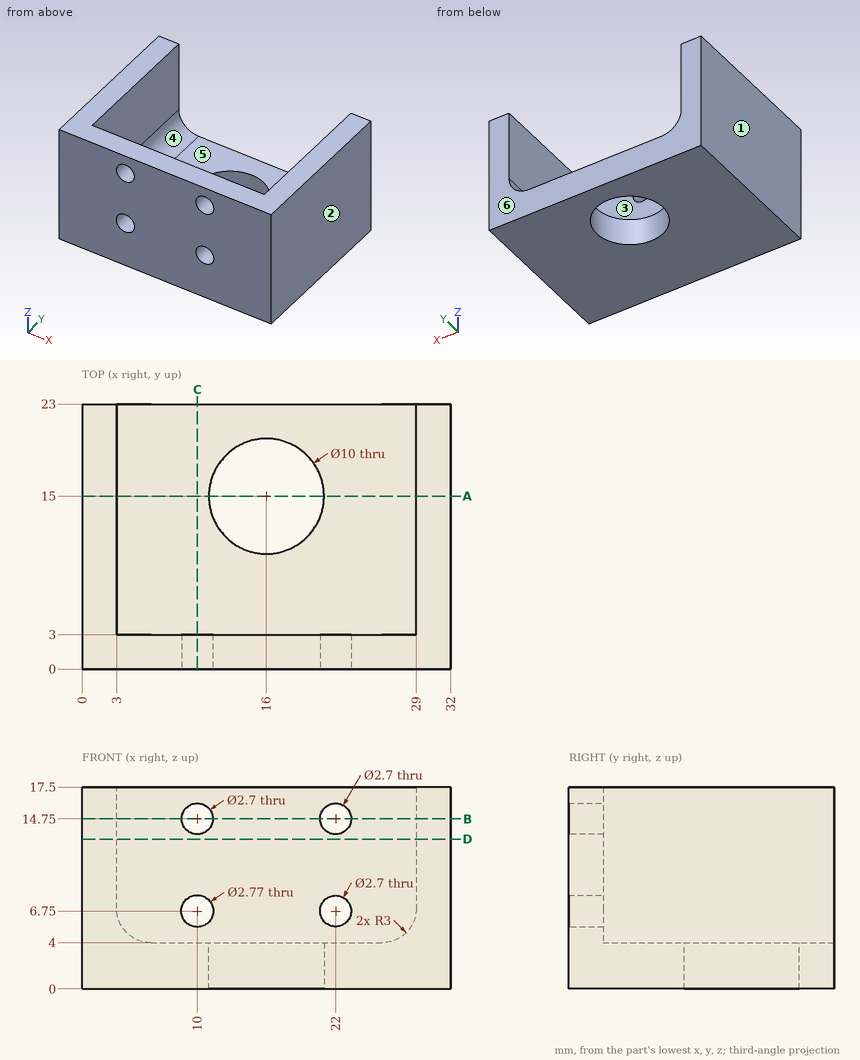
Here's the drawing with two shaded views (mm, measured from the low corner). I have some questions. A direction names the side the tool comes from. Coordinates: 2 decimals unless noted, no trailing zeros. Order: outer loops, then holes, each group sorted by start corner. A loop starts at its lowest first (then second) coordinate and runs counter-clockwise, first axis right, second up.
Item 1: For the marked faces 5 and 6, which set-ups out of +Z, -Z, +X, -X, +Y, -Y let a thin tool reach every point of the face, with its end or its side?
Result sheet:
face 5: +Z, +Y
face 6: +Z, -Z, +X, -X, +Y
Item 2: If we section it at C-C on x = 10: List the corners of the cut face in (y, z) for me (3 decimals), plus the area to 3 significant figures.
Result sheet:
outline: (0, 0) - (23, 0) - (23, 4) - (3, 4) - (3, 5.365) - (0, 5.365) - close; (0, 8.135) - (3, 8.135) - (3, 13.4) - (0, 13.4) - close; (0, 16.1) - (3, 16.1) - (3, 17.5) - (0, 17.5) - close
area: 116 mm2
Item 3: If we section it at B-B on z = 14.75: List the corners of the cut face in (x, y) for me.
Result sheet:
outline: (0, 0) - (8.65, 0) - (8.65, 3) - (3, 3) - (3, 23) - (0, 23) - close; (11.35, 0) - (20.65, 0) - (20.65, 3) - (11.35, 3) - close; (23.35, 0) - (32, 0) - (32, 23) - (29, 23) - (29, 3) - (23.35, 3) - close
Item 4: If we section it at A-A on y = 15: List the corners of the cut face in (x, z) for me.
Result sheet:
outline: (0, 0) - (11, 0) - (11, 4) - (6, 4) arc R3 cw to (3, 7) - (3, 17.5) - (0, 17.5) - close; (21, 0) - (32, 0) - (32, 17.5) - (29, 17.5) - (29, 7) arc R3 cw to (26, 4) - (21, 4) - close
Item 5: For P1, Ø6, axis at x = 16, y = 15, coming from the +Z side; P2, Ø4, axis at x = 21.5, z = 9, coming from the +Y side, each with a flat end and sliding along its axis, tell me the tip position at first contact or that it passes through.
Result sheet:
P1: passes through
P2: stops at y = 3
Item 6: I need wall thicknesses on line 1 (X direction, y = 1.55, z = 14.75); line 2 (X direction, y = 0.85, z = 6.75) (3 decimals); line 3 (X direction, y = 18.25, z = 8.5). Which ranges of each line are inside material? Lowest first, please.
Result sheet:
line 1: x = 0 to 8.65, 11.35 to 20.65, 23.35 to 32
line 2: x = 0 to 8.615, 11.385 to 20.65, 23.35 to 32
line 3: x = 0 to 3, 29 to 32
Item 7: If we mould it in two halves opening along X, with no side actions, what happens to the marked faces 1, 2, 3 and 4? For each: +X half, -X half, draft (parallel to the pull), parting line (faces both ways), or undercut.
Result sheet:
face 1: -X half
face 2: +X half
face 3: undercut
face 4: undercut
Item 8: If we section it at D-D on z = 13: List the corners of the cut face in (x, y) for me, plus the area to 3 significant figures.
Result sheet:
outline: (0, 0) - (32, 0) - (32, 23) - (29, 23) - (29, 3) - (3, 3) - (3, 23) - (0, 23) - close
area: 216 mm2
